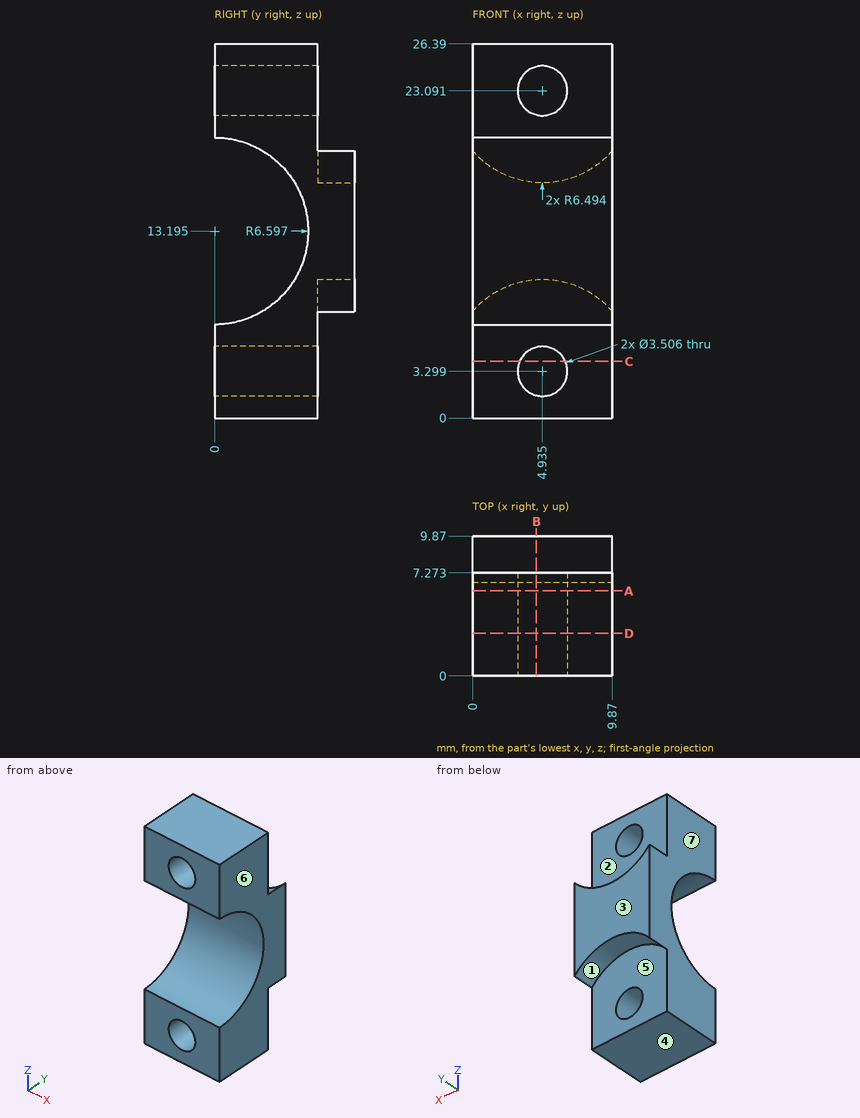
Can you work these out from the drawing? Everything is in mm from the part's minimum corner. A direction names the side the tool comes from. Coordinates: 2 decimals unless noted, no trailing zeros. Loops run counter-clockwise (first coordinate to the right, second up) from the corner with the lowest first, then second, coordinate; pieces in that order, holes last.
1) Imagine slicing it at C-C (z = 4). List the corners of the cut face in (x, y) for me.
Reported:
outline: (0, 0) - (3.33, 0) - (3.33, 7.27) - (0, 7.27) - close; (6.54, 0) - (9.87, 0) - (9.87, 7.27) - (6.54, 7.27) - close
2) Which directions (+Z, -Z, +X, -X, +Y, -Y) give clear straight access to the entire face, cutting with the end or side of a thin tool? Please do the marked faces 1, 2 and 3.
Reported:
face 1: -Z, +Y
face 2: +Z, +Y
face 3: +Z, -Z, +X, -X, +Y
3) Imagine slicing it at D-D (y = 3). List the corners of the cut face in (x, z) for me (1 decimal).
Reported:
outline: (0, 0) - (9.9, 0) - (9.9, 7.3) - (0, 7.3) - close; (0, 19.1) - (9.9, 19.1) - (9.9, 26.4) - (0, 26.4) - close; hole circle Ø3.5 at (4.9, 3.3); hole circle Ø3.5 at (4.9, 23.1)
4) Imagine slicing it at A-A (y = 6). List the corners of the cut face in (x, z) for me (1 decimal), and give its area (3 significant figures).
Reported:
outline: (0, 0) - (9.9, 0) - (9.9, 10.5) - (0, 10.5) - close; (0, 15.9) - (9.9, 15.9) - (9.9, 26.4) - (0, 26.4) - close; hole circle Ø3.5 at (4.9, 3.3); hole circle Ø3.5 at (4.9, 23.1)
area: 187 mm2
5) Will these pins go through, and if not, where does the flat tip stop? pin 1 Ø1.5 at (x, z) = (2, 15.5) entering from -Y; pin 2 Ø5.5 at (x, z) = (4.94, 3.3) entering from +Y.
Reported:
pin 1: stops at y = 5.85
pin 2: stops at y = 7.27
6) Thinking about a two-plate mould opening in X: for the marked faces 4, 5, 6 and 7, which applies, released by +X, released by -X, zero draft, split by the parting line, or undercut?
Reported:
face 4: zero draft
face 5: undercut
face 6: released by +X
face 7: released by -X
7) Please list where these lines run through material, in increasing order: line 1 along Z through (x, y) = (6.5, 3) (1 decimal); line 2 along Z through (x, y) = (6, 2) (1 decimal); line 3 along Z through (x, y) = (5, 8).
Reported:
line 1: z = 0 to 2.5, 4.1 to 7.3, 19.1 to 22.3, 23.9 to 26.4
line 2: z = 0 to 1.9, 4.7 to 6.9, 19.5 to 21.7, 24.5 to 26.4
line 3: z = 9.79 to 16.6
8) Imagine slicing it at B-B (x = 4.5). List the corners of the cut face in (y, z) for me (1 decimal).
Reported:
outline: (0, 0) - (7.3, 0) - (7.3, 1.6) - (0, 1.6) - close; (0, 5) - (7.3, 5) - (7.3, 9.8) - (9.9, 9.8) - (9.9, 16.6) - (7.3, 16.6) - (7.3, 21.4) - (0, 21.4) - (0, 19.8) arc R6.6 cw to (0, 6.6) - close; (0, 24.8) - (7.3, 24.8) - (7.3, 26.4) - (0, 26.4) - close
